The model under review builds one solid part; all positions refer to its coordinate system, in mm. Face numbers are marked on the shaded views. A direction names the side the tool comes from. Coordinates: 2 decimals unless noted, no trailing zeros. Answer in a Markdown table with one row per item. Add a question column.
(1) For line 1 along X through (y, z) = (23.25, 0); line 2 along X through (y, z) = (19, -1); line 3 along Z through (x, y) = (1, 1.5), list the stretches that pass through material, from the lowest coordinate up.
(2) Machinability: for the marked faces 1, 2 and 3, which of the approach directions +Z, -Z, +X, -X, +Y, -Y give a long, thin tool a straight path to every point of the face, cutting with its end or side? Answer none if there is none.
(3) For P1, Ø8.5, axis at x = 0, z = -3, coming from the -Y side; P2, Ø2, axis at x = -4.5, y = 20.5, coming from the -Z side; P3, Ø6, axis at x = 1, z = 6.5, coming from the -Y side; P4, Ø8, axis at x = -1, y = 15, coming from the +Z side, all flat-tipped, find the tip position at first contact; note any pin that passes through.
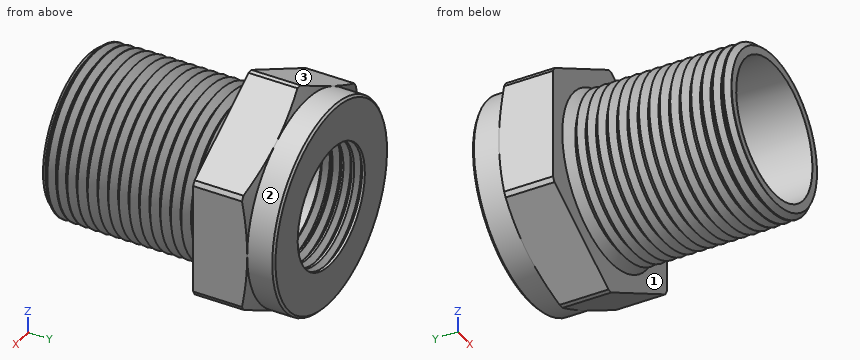
from build123d import *

# Parameters (mm, degrees)
SKETCH2_OUTSIDE_W  = 40.394
SKETCH2_OUTSIDE_H  = 40.394
CUT_EXTRUDE1_DEPTH = 10.906
SKETCH4_OUTSIDE_W  = 43.51
SKETCH4_OUTSIDE_H  = 46.994
SKETCH4_OUTSIDE_R  = 12.446
CUT_EXTRUDE3_DEPTH = 1.27
CUT_EXTRUDE3_DRAFT = -70
CHAMFER2_SIZE      = 0.247603347
CHAMFER2_SIZE2     = 0.254
LPATTERN1_COUNT    = 5
LPATTERN1_PITCH    = 1.27
LPATTERN2_COUNT    = 16
LPATTERN2_PITCH    = 1.27
CHAMFER3_SIZE      = 0.254


with BuildPart() as part:
    # Sketch1 → Revolve1 (revolve)
    with BuildSketch(Plane.XY, mode=Mode.PRIVATE) as revolve1_sk:
        Polygon((8.3312, 0), (9.888553298, 0), (10.414, 20.066), (14.18844, 20.066), (14.18844, 26.65984), (12.446, 26.65984), (12.446, 29.972), (7.342571073, 29.972), (7.2009, 24.5618), (8.281035, 24.5618), (8.281035, 21.5646), (8.3312, 21.5646), align=None)
    revolve(revolve1_sk.sketch.rotate(Axis((0, 0, 0), (0, 1, 0)), 90), axis=Axis((0, 0, 0), (0, 1, 0)))  # turned: the seam where the file's is

    # Sketch2 outside → Cut-Extrude1 (cut, through all)
    with BuildSketch(Plane.XZ.offset(-20.066)):
        Rectangle(SKETCH2_OUTSIDE_W, SKETCH2_OUTSIDE_H)
        Polygon((12.446, 7.18570145), (0, 14.371402901), (-12.446, 7.18570145), (-12.446, -7.18570145), (0, -14.371402901), (12.446, -7.18570145), align=None, mode=Mode.SUBTRACT)
    extrude(amount=-CUT_EXTRUDE1_DEPTH, mode=Mode.SUBTRACT)


with BuildPart() as cut_extrude3_tool:
    # Sketch4 outside → Cut-Extrude3 (with draft: the straight prism first)
    with BuildSketch(Plane(origin=(0, 26.65984, 0), x_dir=(-1, 0, 0), z_dir=(0, 1, 0))):
        Rectangle(SKETCH4_OUTSIDE_W, SKETCH4_OUTSIDE_H)
        with Locations(Location((0, 0, 0), (0, 0, 270))):  # turned: the seam where the file's is
            Circle(SKETCH4_OUTSIDE_R, mode=Mode.SUBTRACT)
    extrude(amount=-CUT_EXTRUDE3_DEPTH)
    # Cut-Extrude3: the draft: its side faces are tilted about the plane it starts from
    cut_extrude3_sides = [cut_extrude3_tool.faces().sort_by_distance(p)[0] for p in [
        (0, 26.02484, -23.497),
        (-21.755, 26.02484, 0),
        (0, 26.02484, 23.497),
        (21.755, 26.02484, 0),
        (0, 26.02484, 12.446),
    ]]
    draft(cut_extrude3_sides, Plane(origin=(0, 26.65984, 0), x_dir=(-1, 0, 0), z_dir=(0, 1, 0)), CUT_EXTRUDE3_DRAFT)


with BuildPart() as part_1:
    add(part.part)

    # Cut-Extrude3: cut by cut_extrude3_tool
    add(cut_extrude3_tool.part, mode=Mode.SUBTRACT)

    # Chamfer2
    chamfer2_edges = [part_1.edges().sort_by_distance(p)[0] for p in [
        (0, 24.5618, 7.2009),
    ]]
    chamfer2_side = [part_1.faces().sort_by_distance(p)[0] for p in [
        (0, 27.2669, 7.271735536),
    ]]
    chamfer(chamfer2_edges, length=CHAMFER2_SIZE, length2=CHAMFER2_SIZE2, reference=chamfer2_side[0])

    # Sketch7 → Cut-Revolve1 (revolve, cut)
    with BuildSketch(Plane.XY, mode=Mode.PRIVATE) as cut_revolve1_sk:
        Polygon((-7.2073815, 24.8093185), (-7.2359604, 25.900702651), (-8.001, 25.334603126), align=None)
    cut_revolve1 = revolve(cut_revolve1_sk.sketch.rotate(Axis((0, 0, 0), (0, 1, 0)), 270), axis=Axis((0, 0, 0), (0, 1, 0)), mode=Mode.SUBTRACT)  # turned: the seam where the file's is

    # LPattern1: Cut-Revolve1 ×5
    with Locations(*[(0, i * LPATTERN1_PITCH, 0) for i in range(1, LPATTERN1_COUNT)]):
        add(cut_revolve1, mode=Mode.SUBTRACT)

    # Sketch8 → Cut-Revolve2 (revolve, cut)
    with BuildSketch(Plane.XY, mode=Mode.PRIVATE) as cut_revolve2_sk:
        Polygon((-10.414, 20.066), (-9.121156991, 19.210285879), (-10.367443587, 18.28808231), align=None)
    cut_revolve2 = revolve(cut_revolve2_sk.sketch.rotate(Axis((0, 0, 0), (0, 1, 0)), 270), axis=Axis((0, 0, 0), (0, 1, 0)), mode=Mode.SUBTRACT)  # turned: the seam where the file's is

    # LPattern2: Cut-Revolve2 ×16
    with Locations(*[(0, -i * LPATTERN2_PITCH, 0) for i in range(1, LPATTERN2_COUNT)]):
        add(cut_revolve2, mode=Mode.SUBTRACT)

    # Chamfer3
    chamfer3_edges = [part_1.edges().sort_by_distance(p)[0] for p in [
        (0, 29.972, 12.446),
    ]]
    chamfer(chamfer3_edges, length=CHAMFER3_SIZE)


solid = part_1.part
Outcome:
| question | item | result |
|---|---|---|
| 1 | line 1 | -12.45 to -8.28, 8.28 to 12.45 |
| 1 | line 2 | -9.35 to -8.27, 8.27 to 9.35 |
| 1 | line 3 | -9.17 to -8.27, 8.27 to 9.17 |
| 2 | face 1 | -Y |
| 2 | face 2 | +Y |
| 2 | face 3 | +Z, -X, +Y, -Y |
| 3 | P1 | y = 24.77 |
| 3 | P2 | z = -12.35 |
| 3 | P3 | y = 0 |
| 3 | P4 | z = 10.03 |
